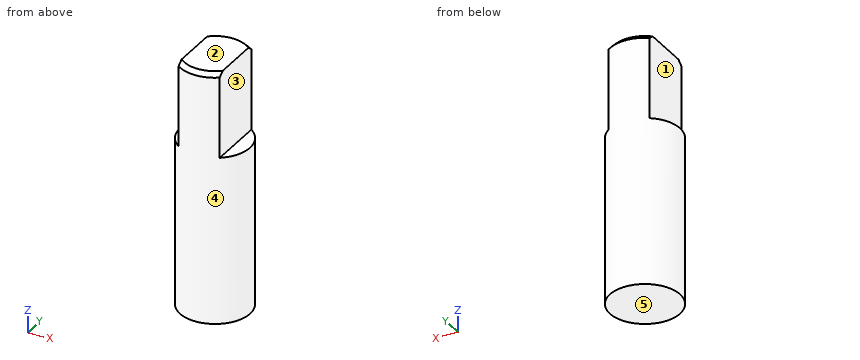
```python
from build123d import *

# Parameters (mm, degrees)
SKETCH1_R           = 2.475
EXTRUDE1_DEPTH      = 17.8
SKETCH2_OUTSIDE_W   = 10.776
SKETCH2_OUTSIDE_H   = 10.776
SKETCH2_OUTSIDE_W_2 = 2.9
SKETCH2_OUTSIDE_H_2 = 7
EXTRUDE2_DEPTH      = 6
CHAMFER1_SIZE       = 0.3


with BuildPart() as part:
    # Sketch1 → Extrude1 (new body)
    with BuildSketch(Plane.XY):
        Circle(SKETCH1_R)
    extrude(amount=EXTRUDE1_DEPTH)

    # Sketch2 outside → Extrude2 (cut)
    with BuildSketch(Plane.XY.offset(17.8)):
        Rectangle(SKETCH2_OUTSIDE_W, SKETCH2_OUTSIDE_H)
        Rectangle(SKETCH2_OUTSIDE_W_2, SKETCH2_OUTSIDE_H_2, mode=Mode.SUBTRACT)
    extrude(amount=-EXTRUDE2_DEPTH, mode=Mode.SUBTRACT)

    # Chamfer1
    chamfer1_edges = [part.edges().sort_by_distance(p)[0] for p in [
        (0, 2.475, 17.8),
        (0, -2.475, 17.8),
    ]]
    chamfer(chamfer1_edges, length=CHAMFER1_SIZE)


solid = part.part
```
The listing builds one solid part. Answer for the finished solid, in the listing's coordinates (mm). Face numbers are marked on the shaded views. A direction names the side the tool comes from. Give positions to 0.01 mm unless a question says otherwise; leave off trailing zeros. Order: outer loops, then holes, each group sorted by start corner. A loop starts at its lowest first (then second) coordinate and runs counter-clockwise, first axis right, second up.
Item 1: The part is cut by section A-A, the plane y = 0. Give the vertices of the cut face in (x, z) (3 decimals), and give its area (3 significant figures).
From the geometry:
outline: (-2.475, 0) - (2.475, 0) - (2.475, 11.8) - (1.45, 11.8) - (1.45, 17.8) - (-1.45, 17.8) - (-1.45, 11.8) - (-2.475, 11.8) - close
area: 75.8 mm2
Item 2: Find the intervals of material crossed by probe 1 along Z at (x, y) = (-1.5, -1.5); probe 2 along X at (y, z) = (-0.65, 13); probe 3 along X at (y, z) = (-1.45, 1.5), in increasing order.
From the geometry:
probe 1: z = 0 to 11.8
probe 2: x = -1.45 to 1.45
probe 3: x = -2.01 to 2.01
Item 3: The part is cut by section C-C, the plane x = -1.9. Give the vertices of the cut face in (y, z), and give its area (3 significant figures).
From the geometry:
outline: (-1.59, 0) - (1.59, 0) - (1.59, 11.8) - (-1.59, 11.8) - close
area: 37.4 mm2
Item 4: Which of the six approach directions +Z, -Z, +X, -X, +Y, -Y give full straight-line access (tool end or side, diameter ignored) to the marked faces 1, 2 and 3?
From the geometry:
face 1: +Z, -X, +Y, -Y
face 2: +Z, +X, -X, +Y, -Y
face 3: +Z, +X, +Y, -Y
Item 5: The part is cut by section D-D, the plane y = -1. Give the vertices of the cut face in (x, z), and give its area (3 significant figures).
From the geometry:
outline: (-2.26, 0) - (2.26, 0) - (2.26, 11.8) - (1.45, 11.8) - (1.45, 17.8) - (-1.45, 17.8) - (-1.45, 11.8) - (-2.26, 11.8) - close
area: 70.8 mm2
Item 6: Given pin 1 Ø2 at (y, z) = (1.5, 2) entering from -X; pin 2 Ø2 at (y, z) = (-1.5, 14.5) entering from +X; pin 3 Ø2 at (x, z) = (1, 12.5) entering from +Y (3 decimals); pin 4 Ø0.8 at (x, y) = (-2, 0) entering from +Z, each flat-ended and moving along its own axis, determine where each tip first touches the part or whether it passes through.
From the geometry:
pin 1: stops at x = -2.42
pin 2: stops at x = 1.45
pin 3: stops at y = 2.475
pin 4: stops at z = 11.8
Item 7: For a pull along Y with two mould halves and no side action, classify the marked faces 4 and 5 as pulls with the +Y half, pulls with the -Y half, needs draft (parallel to the pull), parting line crosses it, or undercut.
From the geometry:
face 4: parting line crosses it
face 5: needs draft
Item 8: The part is cut by section B-B, the plane z = 16.5. Give the vertices of the cut face in (x, y) (3 decimals).
From the geometry:
outline: (-1.45, -2.006) arc R2.475 ccw to (1.45, -2.006) - (1.45, 2.006) arc R2.475 ccw to (-1.45, 2.006) - close
